Work out the finished part from the listing and answer in its coordinate system (mm). Give positions to 0.01 mm unless a question says otherwise; leave off trailing zeros. Order: outer loops, then holes, each group sorted by start corner. A loop starts at its lowest first (then second) coordinate and runs counter-clockwise, first axis right, second up. Notation, with made-up numbers: (5, 78) - (16, 78) arc R25 cw to (16, 115) - close; hole circle Ø1 at (35.25, 22.5). An arc over 180 degrees is marked (long way). Put each result on its own line as item: value.
```python
from build123d import *

# Parameters (mm, degrees)
SKETCH_1_R          = 12.5
EXTRUDE_1_DEPTH     = 194.5
SKETCH_2_R          = 8
CUT_EXTRUDE_1_DEPTH = 349
SKETCH_3_R          = 10
EXTRUDE_2_DEPTH     = 40
SKETCH_4_R          = 2
CUT_EXTRUDE_2_DEPTH = 1000
SKETCH_5_R          = 12.5
SKETCH_5_R_2        = 8
EXTRUDE_4_DEPTH     = 146.5
EXTRUDE_START       = 146.5
SKETCH_7_R          = 11.680413058
SKETCH_7_R_2        = 8
EXTRUDE_7_DEPTH     = 146.5


with BuildPart() as part:
    # 草图1 → 凸台-拉伸1 (new, symmetric)
    with BuildSketch(Plane.XY):
        Circle(SKETCH_1_R)
    extrude(amount=EXTRUDE_1_DEPTH, both=True)

    # 草图2 → 切除-拉伸1 (cut)
    with BuildSketch(Plane.XY.offset(194.5)):
        Circle(SKETCH_2_R)
    extrude(amount=-CUT_EXTRUDE_1_DEPTH, mode=Mode.SUBTRACT)

    # 草图3 → 凸台-拉伸2 (add)
    with BuildSketch(Plane.XY.offset(194.5)):
        Circle(SKETCH_3_R)
    extrude(amount=-EXTRUDE_2_DEPTH)

    # 草图4 → 切除-拉伸2 (cut)
    with BuildSketch(Plane.XY.offset(194.5)):
        with Locations((0, 8)):
            Circle(SKETCH_4_R)
        with Locations((-6.92820323, -4)):
            Circle(SKETCH_4_R)
        with Locations((6.92820323, -4)):
            Circle(SKETCH_4_R)
        Circle(SKETCH_4_R)
    extrude(amount=-CUT_EXTRUDE_2_DEPTH, mode=Mode.SUBTRACT)

    # 草图5 → 凸台-拉伸4 (add)
    with BuildSketch(Plane.XY):
        Circle(SKETCH_5_R)
        with Locations(Location((0, 0, 0), (0, 0, 344.361511563))):
            Circle(SKETCH_5_R_2, mode=Mode.SUBTRACT)
    extrude(amount=-EXTRUDE_4_DEPTH)

    # 草图7 → 凸台-拉伸7 (add)
    with BuildSketch(Plane.XY.offset(EXTRUDE_START)):
        Circle(SKETCH_7_R)
        with Locations(Location((0, 0, 0), (0, 0, 344.361511563))):
            Circle(SKETCH_7_R_2, mode=Mode.SUBTRACT)
    extrude(amount=-EXTRUDE_7_DEPTH)


solid = part.part
```
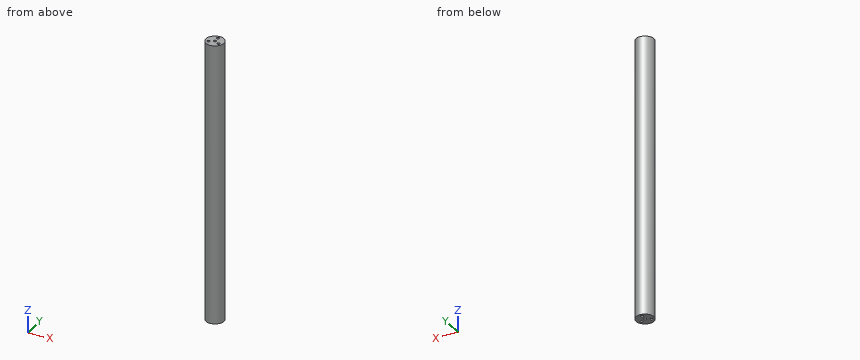
(1) Section A-A, the plane z = -10 is taken. Write down the section's boundary in (x, y).
Geometry check:
outline: circle Ø25 at (0, 0); hole circle Ø16 at (0, 0)
(2) Given pin 1 (2 mm diameter, centred on x = 6.5, z = -53.5, fed in from -Y) (3 decimals); pin 2 (3 mm diameter, centred on x = 0, y = 8, fed in from -Z); pin 3 (2 mm diameter, centred on x = 6, z = -106.5, fed in from -Y), each flat-ended and moving along its own axis, determine where each tip first touches the part or whether it passes through.
Geometry check:
pin 1: stops at y = -11.225
pin 2: stops at z = -146.5
pin 3: stops at y = -11.46
(3) Straight lines are drawn through the part: line 1 (Y direction, x = 0, z = 168); line 2 (X direction, y = 0.75, z = -50); line 3 (X direction, y = -4, z = 181.5). For each, find the intervals that lie inside material, in ascending order.
Geometry check:
line 1: y = -12.5 to -2, 2 to 6, 10 to 12.5
line 2: x = -12.48 to -7.96, 7.96 to 12.48
line 3: x = -11.84 to -8.93, -4.93 to 4.93, 8.93 to 11.84
